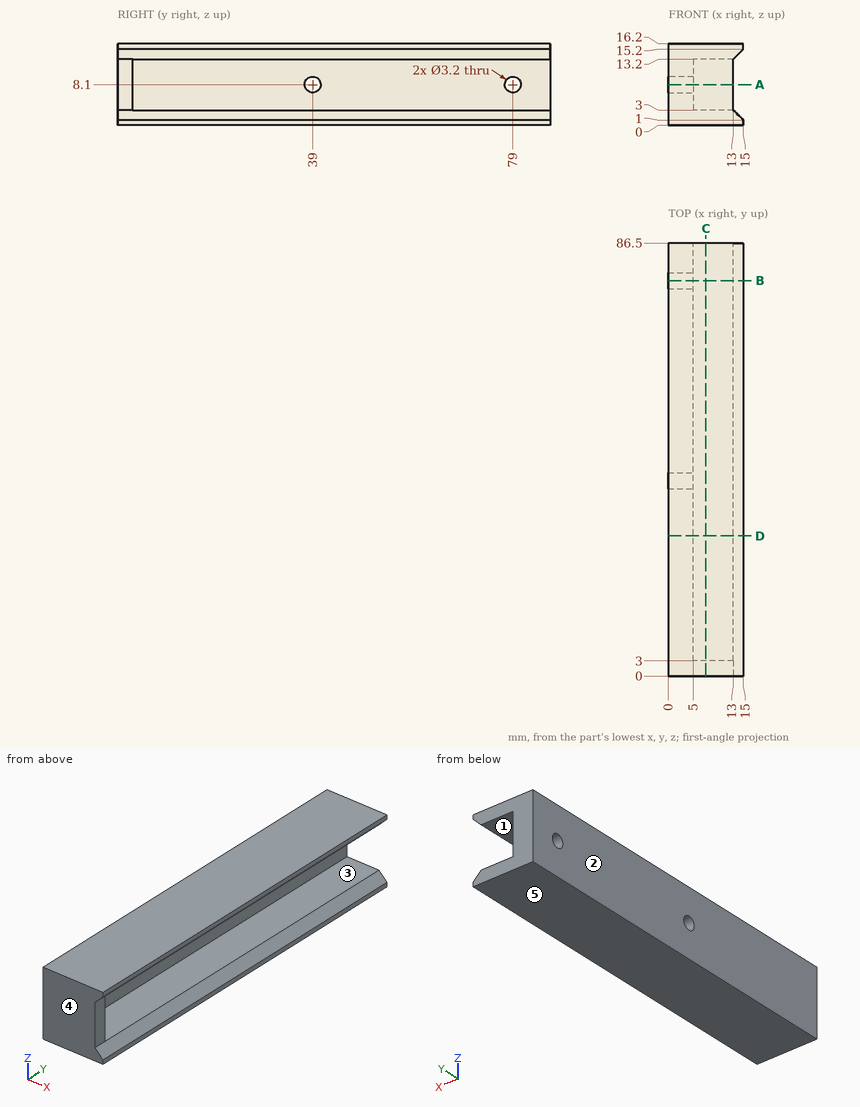
Can you work these out from the drawing? Everything is in mm from the part's minimum corner. A direction names the side the tool comes from. Coordinates: 2 decimals unless noted, no trailing zeros. Loops run counter-clockwise (first coordinate to the right, second up) from the corner with the lowest first, then second, coordinate; pieces in that order, holes last. Notation, with made-up numbers: (42.25, 38) -> (57.25, 38) arc R20 cw to (57.25, 74) -> close; hole circle Ø11 at (45, 72). An arc over 180 degrees is marked (long way). Return JSON: item names as keys, results as strings.
1) Thinking about a two-plate mould opening in Z: for the marked faces 3, 4 and 5, which applies, +Z half, -Z half, draft (parallel to the pull), parting line (faces both ways), or undercut?
Results below:
{"face 3": "undercut", "face 4": "draft", "face 5": "-Z half"}
2) I need wall thicknesses on line 1 (Y direction, x = 2.95, z = 8.1); line 2 (Z direction, x = 1.85, y = 79); line 3 (Z direction, x = 7.25, y = 80.5). Which ranges of each line are inside material? Lowest first, please. Write a range as from..to.
Results below:
{"line 1": "0..37.4, 40.6..77.4, 80.6..86.5", "line 2": "0..6.5, 9.7..16.2", "line 3": "0..3, 13.2..16.2"}
3) If we section it at C-C, the plane x = 7.5: Write out the boundary of the cut face in (y, z).
Results below:
{"outline": "(0, 0) -> (86.5, 0) -> (86.5, 3) -> (3, 3) -> (3, 13.2) -> (86.5, 13.2) -> (86.5, 16.2) -> (0, 16.2) -> close"}
4) For the marked faces 1 and 2, which set-ups out of +Z, -Z, +X, -X, +Y, -Y let a thin tool reach every point of the face, with its end or its side?
Results below:
{"face 1": "+X, +Y", "face 2": "+Z, -Z, -X, +Y, -Y"}
5) Will these pins go through, and if not, where does the flat tip stop? pin 1 (4 mm diameter, centred on y = 39, z = 8.1, fed in from +X); pin 2 (8 mm diameter, centred on y = 55.5, z = 6, fed in from +X); pin 3 (2.5 mm diameter, centred on y = 1, z = 6, fed in from +X).
Results below:
{"pin 1": "x = 5", "pin 2": "x = 14", "pin 3": "x = 13"}
6) If we section it at B-B, the plane y = 79: Write out the boundary of the cut face in (x, z), then the cut area to 3 significant figures.
Results below:
{"outline": "(0, 0) -> (15, 0) -> (15, 1) -> (13, 3) -> (5, 3) -> (5, 6.5) -> (0, 6.5) -> close; (0, 9.7) -> (5, 9.7) -> (5, 13.2) -> (13, 13.2) -> (15, 15.2) -> (15, 16.2) -> (0, 16.2) -> close", "area": "121 mm²"}
7) If we section it at D-D, the plane y = 28: Write out the boundary of the cut face in (x, z), then the cut area to 3 significant figures.
Results below:
{"outline": "(0, 0) -> (15, 0) -> (15, 1) -> (13, 3) -> (5, 3) -> (5, 13.2) -> (13, 13.2) -> (15, 15.2) -> (15, 16.2) -> (0, 16.2) -> close", "area": "137 mm²"}
8) If we section it at A-A, the plane z = 8.1: Write out the boundary of the cut face in (x, y), then the cut area to 4 significant figures.
Results below:
{"outline": "(0, 0) -> (13, 0) -> (13, 3) -> (5, 3) -> (5, 37.4) -> (0, 37.4) -> close; (0, 40.6) -> (5, 40.6) -> (5, 77.4) -> (0, 77.4) -> close; (0, 80.6) -> (5, 80.6) -> (5, 86.5) -> (0, 86.5) -> close", "area": "424.5 mm²"}
